The model under review builds one solid part; all positions refer to its coordinate system, in mm. Face numbers are marked on the shaded views. Coordinates: 2 decimals unless noted, no trailing zeros. Loops run counter-clockwise (first coordinate to the right, second up) from the corner with the lowest first, then second, coordinate; pieces in that order, holes last. Notation, with made-up numbers: (-13.5, 13) - (9.5, 13) arc R32 cw to (9.5, 42) - close; hole circle Ø6 at (70.25, 56.5). An arc over 180 degrees is marked (long way). Answer in a Markdown table with one row per item. Add a question column.
(1) For line 1 along Y through (x, z) = (-4, 4) (3 decimals); line 2 along Z through (x, y) = (-2.75, 4); line 3 along Y through (x, z) = (-4, 5) (3 decimals), list the stretches that pass through material, from the lowest coordinate up.
(2) We need section D-D on z = 1. Write out the cut boundary in (x, y) (3 decimals).
(3) Mouldability with a two-part tool opening along X and no side actions: class the marked faces 1, 2, 3 and 4 as +X half, -X half, draft (parallel to the pull), parting line (faces both ways), or undercut.
(4) We need section C-C on y = 4. Write out the cut boundary in (x, z).
(5) We need section B-B on x = -4. Write out the cut boundary in (y, z) (3 decimals), plus the area to 3 significant figures.
(6) We need section A-A on z = 4. Write out the cut boundary in (x, y) (3 decimals).
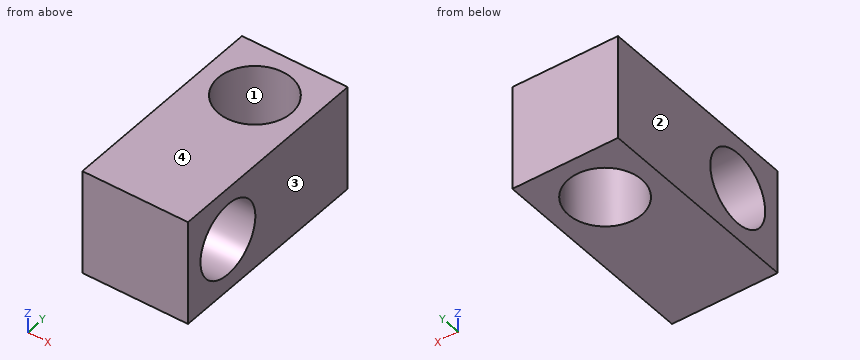
Autodesk Fusion 360 part; units mm, degrees
sketch "スケッチ1" plane through (0, 0, 0) normal (0, 0, 1) x (1, 0, 0)
  line L0 (0, 0) -> (-8, 0)
  line L1 (-8, 0) -> (-8, 16)
  line L2 (-8, 16) -> (0, 16)
  line L3 (0, 16) -> (0, 0)
  dimension "d1" = 8
  dimension "d2" = 16
extrude "押し出し1" add sketch "スケッチ1" along normal blind 8
sketch "スケッチ2" plane through (0, 0, 0) normal (1, 0, 0) x (0, 1, 0)
  line L0 (0, 0) -> (16, 0)
  line L1 (16, 0) -> (16, 8)
  line L2 (16, 8) -> (0, 8)
  line L3 (0, 8) -> (0, 0)
  point P0 (4, 4)
  dimension "d5" = 4
  dimension "d6" = 4
hole "穴1" at (0, 4, 4) direction (-1, 0, 0) diameter 5.5 depth 10 tip angle 118
sketch "スケッチ3" plane through (0, 0, 8) normal (0, 0, 1) x (-1, 0, 0)
  line L0 (0, -16) -> (8, -16)
  line L1 (8, -16) -> (8, 0)
  line L2 (8, 0) -> (0, 0)
  line L3 (0, 0) -> (0, -16)
  point P0 (4, -12)
  dimension "d10" = 4
  dimension "d11" = 4
hole "穴2" at (-4, 12, 8) direction (0, 0, -1) diameter 5.55 depth 10 tip angle 118
Outcome:
| question | item | result |
|---|---|---|
| 1 | line 1 | 0 to 1.25, 6.75 to 9.225, 14.775 to 16 |
| 1 | line 2 | 0 to 1.25, 6.75 to 8 |
| 1 | line 3 | 0 to 1.438, 6.562 to 9.225, 14.775 to 16 |
| 2 | outline | (-8, 0) - (0, 0) - (0, 16) - (-8, 16) - close; hole circle Ø5.55 at (-4, 12) |
| 3 | face 1 | undercut |
| 3 | face 2 | -X half |
| 3 | face 3 | +X half |
| 3 | face 4 | draft |
| 4 | outline | (-8, 0) - (0, 0) - (0, 1.25) - (-8, 1.25) - close; (-8, 6.75) - (0, 6.75) - (0, 8) - (-8, 8) - close |
| 5 | outline | (0, 0) - (9.225, 0) - (9.225, 8) - (0, 8) - close; (14.775, 0) - (16, 0) - (16, 8) - (14.775, 8) - close; hole circle Ø5.5 at (4, 4) |
| 5 | area | 59.8 mm² |
| 6 | outline | (-8, 0) - (0, 0) - (0, 1.25) - (-8, 1.25) - close; (-8, 6.75) - (0, 6.75) - (0, 16) - (-8, 16) - close; hole circle Ø5.55 at (-4, 12) |
